Design review of the part built by this model. Coordinates are the model's own, in mm. Give positions to 0.01 mm unless a question says otherwise; leave off trailing zeros. Loops run counter-clockwise (first coordinate to the right, second up) from the corner with the lowest first, then second, coordinate; pieces in that order, holes last.
Autodesk Inventor part; units mm, degrees
ref_plane "YZ Plane" through (0, 0, 0) normal (1, 0, 0) x (0, 1, 0)
ref_plane "XZ Plane" through (0, 0, 0) normal (0, 1, 0) x (-1, 0, 0)
ref_plane "XY Plane" through (0, 0, 0) normal (0, 0, 1) x (1, 0, 0)
sketch "Sketch1" plane through (0, 0, 0) normal (0, 1, 0) x (-1, 0, 0)
  circle A0 centre (0, 0) radius 6.35
  dimension "d0" = 12.7
extrude "Extrusion1" add sketch "Sketch1" along normal blind 168.275
sketch "Sketch2" plane through (0, 0, 0) normal (0, -1, 0) x (1, 0, 0)
  circle A0 centre (0, 0) radius 3.175
  dimension "d3" = 6.35
extrude "Extrusion2" cut sketch "Sketch2" against normal blind 50.8
sketch "Sketch3" plane through (0, 168.275, 0) normal (0, 1, 0) x (1, 0, 0)
  circle A0 centre (0, 0) radius 3.175
  dimension "d6" = 6.35
extrude "Extrusion3" cut sketch "Sketch3" against normal blind 50.8
thread "Thread1"
properties part number "SHOT_0_003_PivotShaft" material "Aluminum 6061"
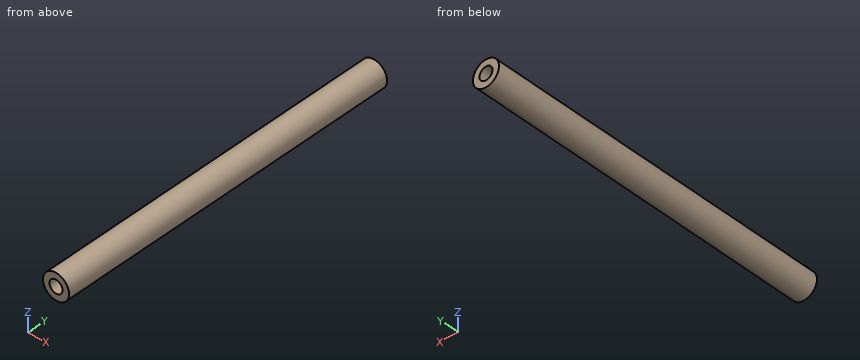
Q1. Take a section at C-C (x = 0). Give the boundary of the cut face in (y, z) (3 decimals), plus the area to 3 significant figures.
Results:
outline: (0, -6.35) - (168.275, -6.35) - (168.275, -3.175) - (117.475, -3.175) - (117.475, 3.175) - (168.275, 3.175) - (168.275, 6.35) - (0, 6.35) - (0, 3.175) - (50.8, 3.175) - (50.8, -3.175) - (0, -3.175) - close
area: 1,490 mm2
Q2. Take a section at A-A (z = 0). Give the boundary of the cut face in (x, y) (3 decimals), plus the area to 3 significant figures.
Results:
outline: (-6.35, 0) - (-3.175, 0) - (-3.175, 50.8) - (3.175, 50.8) - (3.175, 0) - (6.35, 0) - (6.35, 168.275) - (3.175, 168.275) - (3.175, 117.475) - (-3.175, 117.475) - (-3.175, 168.275) - (-6.35, 168.275) - close
area: 1,490 mm2
Q3. Insertion check: pin 1 (1.9 mm diameter, centred on x = 0, z = 1, fed in from -Y); pin 2 (1 mm diameter, centred on y = 115, z = 2.5, fed in from +X); pin 3 (1 mm diameter, centred on y = 119, z = 1, fed in from +X). Each pin has a flat end and moves straight along its axis. Give the tip position at first contact, or say it passes through.
Results:
pin 1: stops at y = 50.8
pin 2: stops at x = 6.03
pin 3: stops at x = 6.33
Q4. Take a section at D-D (y = 71.5). Give the boundary of the cut face in (x, z).
Results:
outline: circle Ø12.7 at (0, 0)
Q5. Take a section at B-B (y = 16.5). Give the boundary of the cut face in (x, z) (3 decimals).
Results:
outline: circle Ø12.7 at (0, 0); hole circle Ø6.35 at (0, 0)
Q6. Wall thickness on line 1 (Z direction, x = 0, y = 142) (3 decimals); line 2 (X direction, y = 85.5, z = 5.5); line 3 (Y direction, x = -1.25, z = 1.75) (3 decimals): over which ranges is each line inside the solid? List them lowest first.
Results:
line 1: z = -6.35 to -3.175, 3.175 to 6.35
line 2: x = -3.17 to 3.17
line 3: y = 50.8 to 117.475
